Model file for the job. Use its own axes, mm. A direction names the side the tool comes from. Give positions to 0.01 mm unless a question says otherwise; leave off trailing zeros. Loops run counter-clockwise (first coordinate to the right, second up) from the corner with the lowest first, then second, coordinate; pieces in that order, holes last. Notation, with made-up numbers: (36.25, 3.5) - (93.25, 3.5) arc R22 cw to (93.25, 22.5) - close; hole circle Ø2 at (-8.75, 27.25). An arc over 180 degrees is marked (long way). Use a Markdown table: item, result.
from build123d import *

# Parameters (mm, degrees)
FILLET1_R = 1
FILLET2_R = 7


with BuildPart() as part:
    # Sketch1 → Revolve1 (revolve)
    with BuildSketch(Plane.XY):
        Polygon((-2.35, 12.482869184), (-3.004199453, 0), (-5.05, 0), (-5.05, -6), (-3.95, -6), (-3.95, -1), (-1.2, -1), (-1.2, 12.482869184), align=None)
    revolve(axis=Axis((0, -1000, 0), (0, 1, 0)))

    # Fillet1
    fillet1_edges = [part.edges().sort_by_distance(p)[0] for p in [
        (2.35, 12.482869184, 0),
        (5.05, 0, 0),
    ]]
    fillet(fillet1_edges, radius=FILLET1_R)

    # Fillet2
    fillet2_edges = [part.edges().sort_by_distance(p)[0] for p in [
        (3.004199453, 0, 0),
    ]]
    fillet(fillet2_edges, radius=FILLET2_R)


solid = part.part
(1) 3-axis set-ups, long thin cutter, end or side, ignore diameter. For faces 4 (the flat face through (-1, -1, 1)), 5 (the cylindrical face through (-4.817, -3.535, 1.517)): which of +Z, -Z, +X, -X, +Y, -Y reach the whole face in a straight line?
Computed:
| item | result |
|---|---|
| face 4 | -Y |
| face 5 | +Y, -Y |
(2) Mould opens along Z. For faces 1 (the conical face through (-2.474, 7.828, 0.779)), 2 (the flat face through (3, -6, -3)), 3 (the cylindrical face through (-0.65, 5.84, 1.01)) say: pulls with the +Z half, pulls with the -Z half, needs draft (parallel to the pull), parting line crosses it, or undercut.
Computed:
| item | result |
|---|---|
| face 1 | parting line crosses it |
| face 2 | needs draft |
| face 3 | undercut |
(3) Pin check, flat tips, straight feed: P1, Ø4, axis at y = 8, z = 0.5, coming from the -X side; P2, Ø2, axis at x = 0, z = 0, coming from the +Y side; P3, Ø2.5, axis at x = 1.5, z = 1.5, coming from the -Y side. Stop position of each tip, or through.
Computed:
| item | result |
|---|---|
| P1 | x = -2.69 |
| P2 | through |
| P3 | y = -1 |
(4) Drill centre lines: probe 1 along Z at (x, y) = (0, 2.75); probe 2 along Z at (x, y) = (2.25, -1.5); probe 3 along X at (y, z) = (-3.75, -1.75). Where is each one in solid material? Low to high. Write a range as [from, to].
Computed:
| item | result |
|---|---|
| probe 1 | [-3.02, -1.2], [1.2, 3.02] |
| probe 2 | [-4.52, -3.25], [3.25, 4.52] |
| probe 3 | [-4.74, -3.54], [3.54, 4.74] |
(5) Slice it at A-A, the plane y = -2. Write the cut outline in (x, z), plus the area to 3 significant figures.
Computed:
| item | result |
|---|---|
| outline | circle Ø10.1 at (0, 0); hole circle Ø7.9 at (0, 0) |
| area | 31.1 mm² |
(6) Slice it at B-B, the plane y = 8. Write the cut outline in (x, z).
Computed:
| item | result |
|---|---|
| outline | circle Ø5.17 at (0, 0); hole circle Ø2.4 at (0, 0) |
